Study the drawing (mm; zero at the part's minimum x, y, z) and answer. A direction names the side the tool comes from. Give positions to 0.01 mm unless a question says otherwise; leave off trailing zeros. Loops run counter-clockwise (first coordinate to the right, second up) from the corner with the lowest first, then second, coordinate; pieces in that order, holes last. Notation, with made-up numbers: (-27.5, 69) - (9.5, 69) arc R19 ccw to (9.5, 95) - close; hole circle Ø4 at (-25.75, 45.5). An arc over 180 degrees is marked (long way). Write item = value, one per line. Start each with the question number.
1) The part is cut by section B-B on x = 11.5. Write down the section's boundary in (y, z) (1 decimal).
2) The part is cut by section C-C on y = 20.5. Write down the section's boundary in (x, z) (1 decimal).
3) The part is cut by section A-A on z = 100. Write down the section's boundary in (x, y) (1 decimal), plus the area to 3 significant figures.
4) Consider probe 1 along Y at (x, z) = (3.5, 100) (1 decimal); probe 2 along Z at (x, y) = (11.25, 53.5); probe 3 along Y at (x, z) = (3, 92) (1 decimal). Determine where each line is inside the solid, lowest interval first.
5) Flat-ended cylindrical pins translate along their axes: P1, Ø2, axis at x = 6, y = 31.5, coming from the -Z side; P2, Ø5, axis at y = 65.875, z = 100, coming from the -X side; P3, Ø5, axis at x = 6.5, z = 29.5, coming from the +Y side (1 decimal); P4, Ø4, axis at x = 12.5, y = 62, coming from the +Z side. Find the tip coordinate at first contact, or state that the pin passes through.
6) Which of the six approach directions +Z, -Z, +X, -X, +Y, -Y give full straight-line access (tool end or side, diameter ignored) to the marked faces 1, 2 and 3?
7) The part is cut by section D-D on z = 65. Write down the section's boundary in (x, y) (1 decimal), plus the area to 3 significant figures.
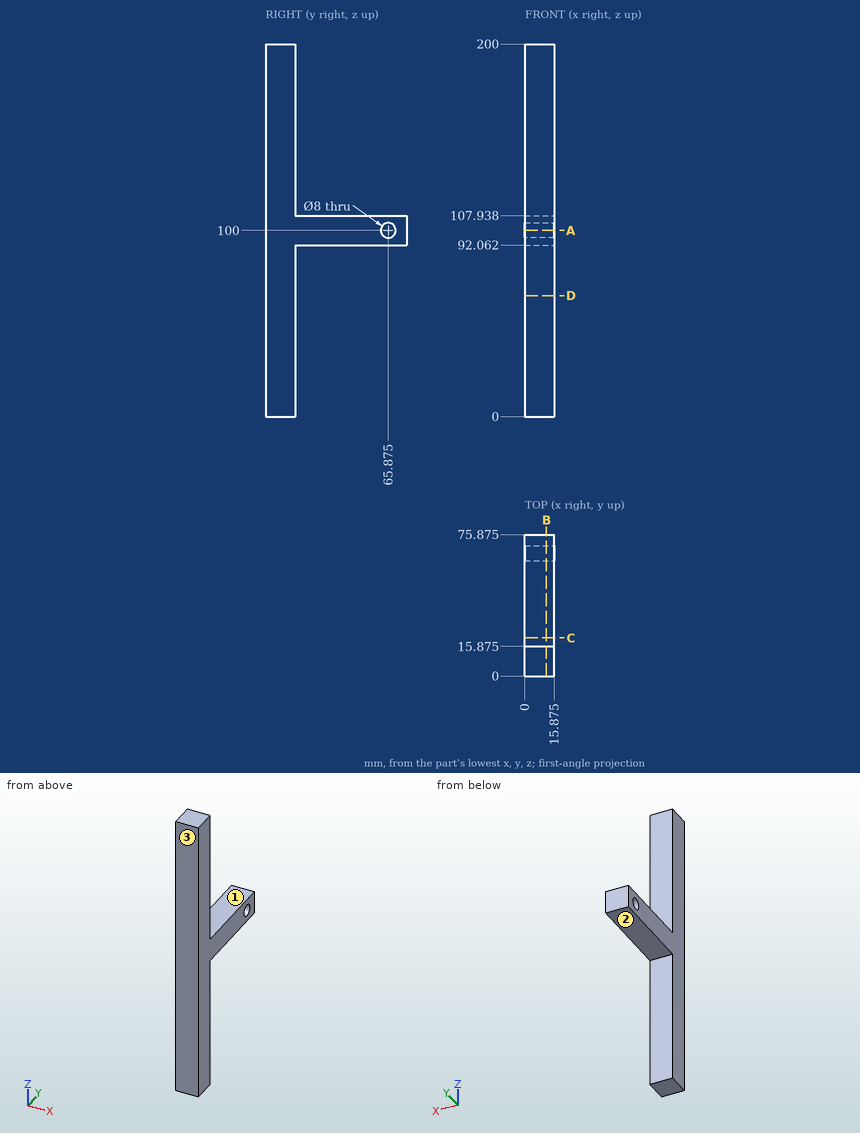
Answer below:
q1.outline = (0, 0) - (15.9, 0) - (15.9, 92.1) - (75.9, 92.1) - (75.9, 107.9) - (15.9, 107.9) - (15.9, 200) - (0, 200) - close; hole circle Ø8 at (65.9, 100)
q2.outline = (0, 92.1) - (15.9, 92.1) - (15.9, 107.9) - (0, 107.9) - close
q3.outline = (0, 0) - (15.9, 0) - (15.9, 61.9) - (0, 61.9) - close; (0, 69.9) - (15.9, 69.9) - (15.9, 75.9) - (0, 75.9) - close
q3.area = 1,080 mm2
q4.probe_1 = 0 to 61.9, 69.9 to 75.9
q4.probe_2 = 92.06 to 107.94
q4.probe_3 = 0 to 15.9
q5.P1 = 92.06
q5.P2 = through
q5.P3 = 15.9
q5.P4 = 107.94
q6.face_1 = +Z, +X, -X, +Y
q6.face_2 = -Z, +X, -X, +Y
q6.face_3 = +Z, -Z, +X, -X, -Y
q7.outline = (0, 0) - (15.9, 0) - (15.9, 15.9) - (0, 15.9) - close
q7.area = 252 mm2
